Autodesk Fusion 360 part; units mm, degrees
sketch "Sketch1" plane through (0, 0, 0) normal (0, 1, 0) x (1, 0, 0)
  line L0 (0, -25) -> (-12.5, -25)
  line L1 (-12.5, -25) -> (12.5, -25)
  line L2 (12.5, -25) -> (37.9, -25)
  circle A0 centre (0, 0) radius 48
  line L3 (37.9, -25) -> (12.5, -25)
  line L4 (12.5, -25) -> (12.5, 0.4)
  line L5 (12.5, 0.4) -> (37.9, 0.4)
  line L6 (37.9, 0.4) -> (37.9, -25)
  line L7 (-12.5, -25) -> (-37.9, -25)
  line L8 (-37.9, -25) -> (-37.9, 0.4)
  line L9 (-37.9, 0.4) -> (-12.5, 0.4)
  line L10 (-12.5, 0.4) -> (-12.5, -25)
  line L11 (-25.2, 0.4) -> (-25.2, -12.3)
  line L12 (12.5, 0.4) -> (25.2, 0.4)
  line L13 (25.2, 0.4) -> (25.2, -12.3)
  line L14 (-25.2, -12.3) -> (25.2, -12.3)
  line L15 (0, -12.3) -> (0, 31.347)
  line L16 (0, 31.347) -> (-25.2, -12.3)
  line L17 (25.2, -12.3) -> (0, 31.347)
  line L18 (0, 31.347) -> (0, 18.647)
  line L19 (0, 18.647) -> (12.7, 18.647)
  line L20 (12.7, 18.647) -> (-12.7, 18.647)
  line L21 (-12.7, 18.647) -> (-12.7, 44.047)
  line L22 (-12.7, 44.047) -> (12.7, 44.047)
  line L23 (12.7, 44.047) -> (12.7, 18.647)
  dimension "d2" = 12.5
  dimension "d3" = 25
  dimension "d4" = 25.4
  dimension "d5" = 96
  dimension "d6" = 25.4
  dimension "d7" = 25.4
  dimension "d8" = 25.4
  dimension "d9" = 25.4
  dimension "d10" = 12.7
  dimension "d11" = 12.7
  dimension "d12" = 12.7
  dimension "d13" = 43.647
  dimension "d14" = 12.7
  dimension "d15" = 12.7
  dimension "d16" = 25.4
  dimension "d17" = 25.4
extrude "Extrude1" add sketch "Sketch1" along normal blind 3 contours L0 L1 L4 L10 L14 | L9 L10 L14 L15 L16 L20 | L4 L5 L12 L14 L15 L17 L19 L20 | A0
extrude "Extrude2" add sketch "Sketch1" along normal blind 1.5 contours L7 L8 L9 L10 L11 L14 | L2 L3 L4 L5 L6 L13 L14 | L9 L10 L14 L16 | L4 L5 L12 L14 L17 | L9 L11 L16 | L5 L12 L13 L17 | L15 L16 L18 L20 | L15 L17 L18 L19 L20 | L16 L17 L19 L20 L21 L22 L23
sketch "Sketch2" plane through (0, 3, 0) normal (0, 1, 0) x (-1, 0, 0)
  line L0 (-12.5, 25) -> (-12.5, -0.4)
  line L1 (-12.5, -0.4) -> (-37.9, -0.4)
  line L2 (-37.9, -0.4) -> (-37.9, 25)
  line L3 (-37.9, 25) -> (-12.5, 25)
  line L4 (12.7, -44.047) -> (-12.7, -44.047)
  line L5 (-12.7, -44.047) -> (-12.7, -18.647)
  line L6 (-12.7, -18.647) -> (12.7, -18.647)
  line L7 (12.7, -18.647) -> (12.7, -44.047)
  line L8 (37.9, -0.4) -> (12.5, -0.4)
  line L9 (12.5, -0.4) -> (12.5, 25)
  line L10 (12.5, 25) -> (37.9, 25)
  line L11 (37.9, 25) -> (37.9, -0.4)
  circle A0 centre (0, 0) radius 48
  line L12 (0, -31) -> (0, -1.902)
  circle A1 centre (0, -1.902) radius 10.5
  line L13 (0, -1.902) -> (0, -7.902)
  line L14 (0, -1.902) -> (-5.1962, 1.098)
  line L15 (0, -1.902) -> (5.1962, 1.098)
  line L16 (0, -1.902) -> (6, -1.902) construction
  circle A2 centre (0, -7.902) radius 2.35
  circle A3 centre (5.1962, 1.098) radius 2.35
  circle A4 centre (-5.1962, 1.098) radius 2.35
  dimension "d22" = 29.098
  dimension "d23" = 21
  dimension "d24" = 6
  dimension "d25" = 60
  dimension "d26" = 6
  dimension "d27" = 30
  dimension "d28" = 6
  dimension "d29" = 4.7
  dimension "d30" = 4.7
  dimension "d31" = 4.7
extrude "Extrude3" add sketch "Sketch2" along normal blind 22 contours A4 | A3 | L12 L13 A2 | L12 L13 A2
Here's how the part is built. I have some questions about the finished solid (model axes, mm). A direction names the side the tool comes from. Round coordinates to 2 decimals unless told otherwise and drop trailing zeros. Loops run counter-clockwise (first coordinate to the right, second up) from the corner with the lowest first, then second, coordinate; pieces in that order, holes last.
1. Thinking about a two-plate mould opening in Z: for faces 1 (the face through (-1, 3, -1)), 2 (the face through (-3.331, 13.846, 2.528)), 3 (the face through (0, 1.5, -32)), which applies, released by +Z, released by -Z, zero draft, split by the parting line, or undercut?
Answers:
face 1: zero draft
face 2: split by the parting line
face 3: undercut
2. Will these pins go through, and if not, where does the flat tip stop? pin 1 (12.5 mm diameter, centred on x = -31.5, z = 15.5, fed in from +Y); pin 2 (1.6 mm diameter, centred on x = -23.5, y = 2.5, fed in from -Z); pin 3 (20.5 mm diameter, centred on x = -5, z = -25.5, fed in from +Y); pin 4 (4 mm diameter, centred on x = -11.5, y = 8, fed in from +Z).
Answers:
pin 1: stops at y = 1.5
pin 2: stops at z = -42.29
pin 3: stops at y = 3
pin 4: passes through
3. Suppose I cut it at B-B, the plane z = 8. Please give me the cut outline in (x, y).
Answers:
outline: (-47.33, 0) - (47.33, 0) - (47.33, 3) - (37.9, 3) - (37.9, 1.5) - (12.5, 1.5) - (12.5, 3) - (-12.5, 3) - (-12.5, 1.5) - (-37.9, 1.5) - (-37.9, 3) - (-47.33, 3) - close
4. Suppose I cut it at A-A, the plane x = 0. Please give me the cut outline in (y, z).
Answers:
outline: (0, -48) - (3, -48) - (3, -44.05) - (1.5, -44.05) - (1.5, -18.65) - (3, -18.65) - (3, -10.25) - (25, -10.25) - (25, -5.55) - (3, -5.55) - (3, 48) - (0, 48) - close
5. Suppose I cut it at D-D, the plane x = 34. Please give me the cut outline in (y, z).
Answers:
outline: (0, -33.88) - (3, -33.88) - (3, -0.4) - (1.5, -0.4) - (1.5, 25) - (3, 25) - (3, 33.88) - (0, 33.88) - close
6. For faces 4 (the face through (0.51, 13.85, -5.61)), 5 (the face through (-5, 25, 1)), which set-ups out of +Z, -Z, +X, -X, +Y, -Y let a thin tool reach every point of the face, with its end or its side?
Answers:
face 4: +Y
face 5: +Z, -Z, +X, -X, +Y
7. If I drill on probe 1 along Y at (x, z) = (-24, -12); probe 2 along Y at (x, z) = (21.5, 21.5); probe 3 along X at (y, z) = (2, -26), over which ranges is the centre line in solid material (lowest first)?
Answers:
probe 1: y = 0 to 3
probe 2: y = 0 to 1.5
probe 3: x = -40.35 to -12.7, 12.7 to 40.35
8. Suppose I cut it at C-C, the plane y = 18.5. Please give me the cut outline in (x, z).
Answers:
outline: circle Ø4.7 at (-5.2, 1.1); circle Ø4.7 at (0, -7.9); circle Ø4.7 at (5.2, 1.1)
